Can you work these out from the model? Positions are in its coordinate system, mm. Face numbers are marked on the shaded views. Round coordinates to 2 decimals unless told otherwise and drop trailing zeros. Loops run counter-clockwise (first coordinate to the right, second up) from the corner with the lowest first, then second, coordinate; pieces in that order, holes last. Notation, with made-up numbers: M 45,22.25 L 53,22.25 A25 ccw 53,37.25 Z; hole C 84.25,4.5 d2. An arc over 180 degrees is marked long. Use a Markdown table: item, result. Add a question column.
```python
from build123d import *

# Parameters (mm, degrees)
ESQUISSE1_W                  = 140
ESQUISSE1_H                  = 75
BOSS_EXTRU_1_DEPTH           = 4.75
ESQUISSE2_R                  = 30.99
ESQUISSE2_R_2                = 27.01
BOSS_EXTRU_2_DEPTH           = 0.25
ENL_V_MAT_EXTRU_1_DEPTH      = 159.894815837
ENL_V_MAT_EXTRU_1_DEPTH_BACK = 159.894815837
ESQUISSE3_R                  = 2
ESQUISSE3_R_2                = 4
ESQUISSE3_R_3                = 1.05


with BuildPart() as part:
    # Esquisse1 → Boss.-Extru.1 (new body)
    with BuildSketch(Plane.XY):
        with Locations((70, 37.5)):
            Rectangle(ESQUISSE1_W, ESQUISSE1_H)
    extrude(amount=BOSS_EXTRU_1_DEPTH)

    # Esquisse2 → Boss.-Extru.2 (add)
    # profile 1 of 2: a face of its own
    with BuildSketch(Plane.XY.offset(4.75)):
        with Locations(Location((35, 37.5, 0), (0, 0, 180))):
            Circle(ESQUISSE2_R)
        with Locations((35, 37.5)):
            Circle(ESQUISSE2_R_2, mode=Mode.SUBTRACT)
    # profile 2 of 2: a face of its own
    with BuildSketch(Plane.XY.offset(4.75)):
        with Locations(Location((105, 37.5, 0), (0, 0, 180))):
            Circle(ESQUISSE2_R)
        with Locations(Location((105, 37.5, 0), (0, 0, 180))):
            Circle(ESQUISSE2_R_2, mode=Mode.SUBTRACT)
    extrude(amount=BOSS_EXTRU_2_DEPTH)

    # Esquisse3 → Enlèv. mat.-Extru.1 (cut, two sides: drawn at the far end of the back side and taken through both)
    with BuildSketch(Plane.XY.offset(4.75).offset(-ENL_V_MAT_EXTRU_1_DEPTH_BACK)):
        with Locations((10, 67.5)):
            Circle(ESQUISSE3_R)
        with Locations((60, 67.5)):
            Circle(ESQUISSE3_R)
        with Locations(Location((60, 7.5, 0), (0, 0, 180))):
            Circle(ESQUISSE3_R)
        with Locations(Location((10, 7.5, 0), (0, 0, 180))):
            Circle(ESQUISSE3_R)
        with Locations((130, 7.5)):
            Circle(ESQUISSE3_R)
        with Locations((80, 7.5)):
            Circle(ESQUISSE3_R)
        with Locations(Location((80, 67.5, 0), (0, 0, 180))):
            Circle(ESQUISSE3_R)
        with Locations(Location((130, 67.5, 0), (0, 0, 180))):
            Circle(ESQUISSE3_R)
        with Locations((35, 37.5)):
            Circle(ESQUISSE3_R_2)
        with Locations((105, 37.5)):
            Circle(ESQUISSE3_R_2)
        with Locations((16.43465241, 59.778417108)):
            Circle(ESQUISSE3_R_3)
        with Locations(Location((53.56534759, 15.221582892, 0), (0, 0, 180))):
            Circle(ESQUISSE3_R_3)
        with Locations(Location((123.56534759, 59.778417108, 0), (0, 0, 180))):
            Circle(ESQUISSE3_R_3)
        with Locations((86.43465241, 15.221582892)):
            Circle(ESQUISSE3_R_3)
    extrude(amount=ENL_V_MAT_EXTRU_1_DEPTH + ENL_V_MAT_EXTRU_1_DEPTH_BACK, mode=Mode.SUBTRACT)


solid = part.part
```
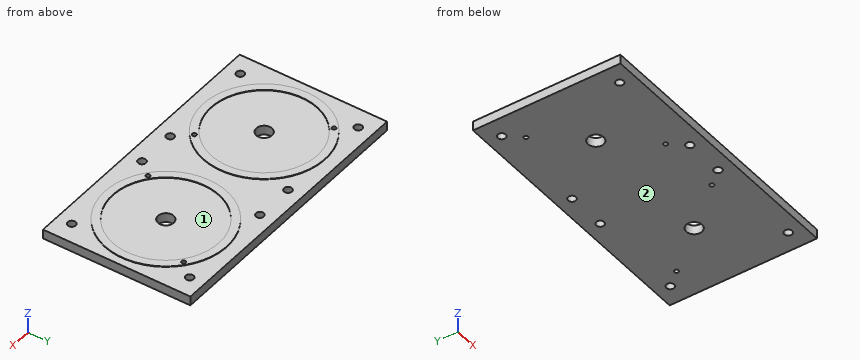
(1) I'm going to push flat-ended pins straight in: pin 1 (1.7 mm diameter, centred on x = 16.43, y = 59.78, fed in from -Z); pin 2 (13 mm diameter, centred on x = 105, y = 37.5, fed in from +Z). Where does each tip first touch, or does it pass through?
(2) Suppose I cut it at A-A on y = 37.5. List the corners of the cut face in (x, z) for me, and give its area (3 significant figures).
(3) Thinking about a two-plate mould opening in X: for the marked faces 1 and 2, which applies, released by +X, released by -X, zero draft, split by the parting line, or undercut?
(4) If I drill on probe 1 along X at (y, z) = (67.5, 1.7); probe 2 along Y at (x, z) = (130, 3.5); probe 3 along Y at (x, z) = (79, 3.15), over which ranges is the centre line in solid material (lowest first)? Write a range as [from, to].
(5) Suppose I cut it at C-C on x = 10. List the corners of the cut face in (y, z) for me, and give its area (3 significant figures).
(6) Suppose I cut it at B-B on x = 105. List the corners of the cut face in (y, z) for me.
(7) Suppose I cut it at D-D on z = 1.5. Count the separate pieces of the cut face and the enclosed holes in it, and give its area (3 significant figures).
Results below:
| question | item | result |
|---|---|---|
| 1 | pin 1 | passes through |
| 1 | pin 2 | stops at z = 4.75 |
| 2 | outline | M 0,0 L 31,0 L 31,4.75 L 7.99,4.75 L 7.99,5 L 4.01,5 L 4.01,4.75 L 0,4.75 Z; M 39,0 L 101,0 L 101,4.75 L 77.99,4.75 L 77.99,5 L 74.01,5 L 74.01,4.75 L 65.99,4.75 L 65.99,5 L 62.01,5 L 62.01,4.75 L 39,4.75 Z; M 109,0 L 140,0 L 140,4.75 L 135.99,4.75 L 135.99,5 L 132.01,5 L 132.01,4.75 L 109,4.75 Z |
| 2 | area | 593 mm² |
| 3 | face 1 | undercut |
| 3 | face 2 | zero draft |
| 4 | probe 1 | x = [0, 8], [12, 58], [62, 78], [82, 128], [132, 140] |
| 4 | probe 2 | y = [0, 5.5], [9.5, 65.5], [69.5, 75] |
| 4 | probe 3 | y = [0, 5.77], [9.23, 65.77], [69.23, 75] |
| 5 | outline | M 0,0 L 5.5,0 L 5.5,4.75 L 0,4.75 Z; M 9.5,0 L 65.5,0 L 65.5,4.75 L 55.81,4.75 L 55.81,5 L 47.72,5 L 47.72,4.75 L 27.28,4.75 L 27.28,5 L 19.19,5 L 19.19,4.75 L 9.5,4.75 Z; M 69.5,0 L 75,0 L 75,4.75 L 69.5,4.75 Z |
| 5 | area | 322 mm² |
| 6 | outline | M 0,0 L 33.5,0 L 33.5,4.75 L 10.49,4.75 L 10.49,5 L 6.51,5 L 6.51,4.75 L 0,4.75 Z; M 41.5,0 L 75,0 L 75,4.75 L 68.49,4.75 L 68.49,5 L 64.51,5 L 64.51,4.75 L 41.5,4.75 Z |
| 7 | separate pieces | 1 |
| 7 | enclosed holes | 14 |
| 7 | area | 10,300 mm² |
